Design review of the part built by this model. Coordinates are the model's own, in mm. Face numbers are marked on the shaded views. Round coordinates to 2 decimals unless told otherwise and drop trailing zeros. Order: outer loops, then holes, each group sorted by start corner. A loop starts at its lowest first (then second) coordinate and runs counter-clockwise, first axis right, second up.
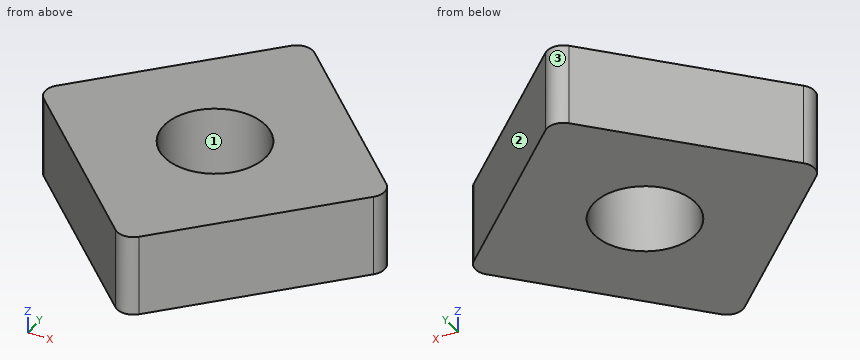
Autodesk Inventor part; units mm, degrees
ref_plane "YZ Plane" through (0, 0, 0) normal (1, 0, 0) x (0, 1, 0)
ref_plane "XZ Plane" through (0, 0, 0) normal (0, 1, 0) x (-1, 0, 0)
ref_plane "XY Plane" through (0, 0, 0) normal (0, 0, 1) x (1, 0, 0)
ref_plane "Arbeitsebene1" through (0, 0, 0) normal (0, 0, 1) x (1, 0, 0)
sketch "Skizze1" plane through (0, 0, 0) normal (0, 0, 1) x (1, 0, 0)
  circle A0 centre (-5.0971, -17.293) radius 1.4
  circle A1 centre (-17.4192, -5.2278) radius 1.4
  arc A2 (5.6957, 26.2674) -> (7.9686, 25.6694) centre (6.0612, 23.038) ccw
  arc A3 (5.6957, 26.2674) -> (-18.8161, -19.193) centre (0, 0) ccw
  arc A4 (-18.1702, -19.8055) -> (-18.8161, -19.193) centre (-16.2778, -17.1634) ccw
  arc A5 (-18.1702, -19.8055) -> (25.9554, 6.9811) centre (0, 0) ccw
  arc A6 (25.2463, 9.2218) -> (25.9554, 6.9811) centre (22.7119, 7.1872) ccw
  arc A7 (25.2463, 9.2218) -> (7.9686, 25.6694) centre (0, 0) ccw
  spline S0 degree 3 poles (-11.5553, -6.2972) (-11.3711, -6.4814) (-11.2247, -6.6998) (-11.0238, -7.1803) (-10.9713, -7.4379) (-10.9679, -7.9586) (-11.0171, -8.2168) (-11.2083, -8.6915) (-11.3454, -8.905) (-11.5184, -9.0874) knots 0 0 0 0 0.252225 0.252225 0.504373 0.504373 0.756494 0.756494 1 1 1 1
  line L0 (-11.5553, -6.2972) -> (-16.3497, -1.5028)
  arc A8 (-16.3497, 1.4985) -> (-16.3497, -1.5028) centre (-14.8491, -0.0022) ccw
  line L1 (-16.3497, 1.4985) -> (-1.5005, 16.3477)
  arc A9 (1.5007, 16.3477) -> (-1.5005, 16.3477) centre (0.0001, 14.8471) ccw
  line L2 (1.5007, 16.3477) -> (16.35, 1.4985)
  arc A10 (16.35, -1.5028) -> (16.35, 1.4985) centre (14.8494, -0.0022) ccw
  line L3 (16.35, -1.5028) -> (1.5007, -16.352)
  arc A11 (-1.5005, -16.352) -> (1.5007, -16.352) centre (0.0001, -14.8514) ccw
  line L4 (-1.5005, -16.352) -> (-4.7949, -13.0576)
  spline S1 degree 3 poles (-7.585, -13.0208) (-7.3961, -12.8415) (-7.1739, -12.7009) (-6.6882, -12.5128) (-6.4293, -12.4671) (-5.9087, -12.4775) (-5.6519, -12.5335) (-5.1824, -12.7372) (-4.9727, -12.8798) (-4.7949, -13.0576) knots 0 0 0 0 0.252231 0.252231 0.504388 0.504388 0.756517 0.756517 1 1 1 1
  arc A12 (-11.5184, -9.0874) -> (-7.585, -13.0208) centre (-9.4998, -11.0022) ccw
  line L5 (-4.7949, -13.0576) -> (-11.5553, -6.2972)
  line L6 (-15.9962, -1.1492) -> (-11.2017, -5.9437)
  arc A13 (-11.1557, -9.4315) -> (-7.9291, -12.658) centre (-9.4998, -11.0022) ccw
  line L7 (-4.4413, -12.7041) -> (-1.1469, -15.9985)
  arc A14 (-1.1469, -15.9985) -> (1.1472, -15.9985) centre (0.0001, -14.8514) ccw
  line L8 (1.1472, -15.9985) -> (15.9964, -1.1492)
  arc A15 (15.9964, -1.1492) -> (15.9964, 1.1449) centre (14.8494, -0.0022) ccw
  line L9 (15.9964, 1.1449) -> (1.1472, 15.9941)
  arc A16 (1.1472, 15.9941) -> (-1.1469, 15.9941) centre (0.0001, 14.8471) ccw
  line L10 (-1.1469, 15.9941) -> (-15.9962, 1.1449)
  arc A17 (-15.9962, 1.1449) -> (-15.9962, -1.1492) centre (-14.8491, -0.0022) ccw
  line L11 (-4.4414, -12.704) -> (-11.2017, -5.9437)
  circle A18 centre (0, 0) radius 5
  spline S2 degree 5 poles (-11.2017, -5.9437) (-10.656, -6.4897) (-10.3193, -7.2462) (-10.3079, -8.1062) (-10.6246, -8.8713) (-11.1557, -9.4315) knots 0 0 0 0 0 0 1 1 1 1 1 1
  spline S3 degree 5 poles (-7.9291, -12.658) (-7.3689, -12.1269) (-6.6038, -11.8103) (-5.7438, -11.8216) (-4.9873, -12.1584) (-4.4413, -12.7041) knots 0 0 0 0 0 0 1 1 1 1 1 1
  point P0 (0, 0)
  dimension "d0" = 0.5
  dimension "d1" = 10
extrude "Extrusion1" add sketch "Skizze1" along normal blind 8 contours L6 A17 L10 A16 L9 A15 L8 A14 L7 L11
properties part number "IM_Matchboxscope_lightdiffusor"
1) To check wall thickness, follow line 1 along Y through (x, z) = (0, 3.25); line 2 along Y through (x, z) = (1, 3.5); line 3 along X through (y, z) = (2, 1.75). State the ranges of each line that lie inside material, in increasing order.
Results:
line 1: y = -16.47 to -5, 5 to 16.47
line 2: y = -16.13 to -4.9, 4.9 to 16.12
line 3: x = -15.14 to -4.58, 4.58 to 15.14
2) Take a section at B-B on z = 2.75. Give the boundary of the cut face in (x, y), plus the area to 3 significant figures.
Results:
outline: (-16, -1.15) - (-1.15, -16) arc R1.62 ccw to (1.15, -16) - (16, -1.15) arc R1.62 ccw to (16, 1.14) - (1.15, 15.99) arc R1.62 ccw to (-1.15, 15.99) - (-16, 1.14) arc R1.62 ccw to start; hole circle Ø10 at (0, 0)
area: 507 mm2
3) Take a section at D-D on y = -7. Give the boundary of the cut face in (x, z).
Results:
outline: (-10.15, 0) - (10.15, 0) - (10.15, 8) - (-10.15, 8) - close
4) Clearance check with flat-ended pins moving along their axes: P1, Ø1.5, axis at x = 4.5, z = 6.5, coming from the -Y side; P2, Ø4, axis at y = -9, z = 5.5, coming from the +X side; P3, Ø2, axis at x = 9.5, z = 7, coming from the +Y side. State where each tip first meets the part, or that it passes through.
Results:
P1: stops at y = -13.4
P2: stops at x = 10.15
P3: stops at y = 8.64
5) Take a section at A-A on y = 0. Give the boundary of the cut face in (x, z).
Results:
outline: (-16.47, 0) - (-5, 0) - (-5, 8) - (-16.47, 8) - close; (5, 0) - (16.47, 0) - (16.47, 8) - (5, 8) - close
6) The part is to be moulded in two halves that separate along X. For the marked faces 1, 2 and 3, say which applies: released by +X, released by -X, zero draft, split by the parting line, or undercut.
Results:
face 1: undercut
face 2: released by +X
face 3: split by the parting line
